Geometry: final body of the model. Coordinates: model frame, mm. Give positions to 0.01 mm unless a question says otherwise; leave off trailing zeros. Order: outer loops, then holes, each group sorted by start corner. A loop starts at its lowest first (then second) coordinate and runs counter-clockwise, first axis right, second up. Notation, with made-up numbers: (17.5, 18.5) - (57.5, 18.5) arc R4 ccw to (57.5, 23.5) - close; hole circle Ø11 at (63, 22). An arc over 180 degrees is marked (long way). Put each result on its own line as item: value. Start each with the question number.
1. Section D-D on z = 3.8. Return the cut outline in (x, y).
2. Ray query, line 1 along Y through (x, z) = (-8.25, 6.6); line 2 along Z through (x, y) = (-6.5, 2.75); line 3 along X through (y, z) = (1.5, 4.55). Return the intervals inside material, ascending. Write a range as from..to.
3. Section A-A on y = 3. Return the cut outline in (x, z).
4. Section B-B on z = 6.6. Return the cut outline in (x, y).
5. Section C-C on x = -7.5. Return the cut outline in (y, z), plus the area to 3 significant figures.
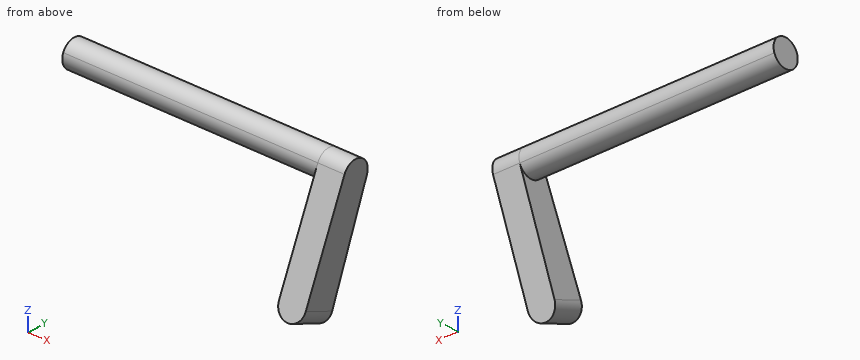
Autodesk Inventor part; units mm, degrees
ref_plane "YZ Plane" through (0, 0, 0) normal (1, 0, 0) x (0, 1, 0)
ref_plane "XZ Plane" through (0, 0, 0) normal (0, 1, 0) x (-1, 0, 0)
ref_plane "XY Plane" through (0, 0, 0) normal (0, 0, 1) x (1, 0, 0)
sketch "Sketch1" plane through (0, 0, 0) normal (1, 0, 0) x (0, 1, 0)
  line L0 (0, 0) -> (2.696, 0)
  line L1 (2.696, 0) -> (2.696, 6.6)
  circle A0 centre (2.696, 6.6) radius 0.5
  line L2 (-0.5, 0.5) -> (0.5, 0.5)
  line L3 (0.5, 0.5) -> (0.5, -0.5)
  line L4 (0.5, -0.5) -> (-0.5, -0.5)
  line L5 (-0.5, -0.5) -> (-0.5, 0.5)
  line L6 (-0.5, 0.5) -> (0.5, -0.5) construction
  line L7 (0.5, 0.5) -> (-0.5, -0.5) construction
  line L8 (0.5, -0.5) -> (3.1627, 6.4205)
  line L9 (-0.5, 0.5) -> (2.2374, 6.7993)
  dimension "d0" = 2.696
  dimension "d1" = 6.6
  dimension "d2" = 1
  dimension "d3" = 1
  dimension "d4" = 1
extrude "Extrusion1" add sketch "Sketch1" along normal blind 1 contours L3 L2 L9 A0 L1 L8 L0 | L3 L4 L5 L2 | L0 L8 L3 | L1 A0 L8 | A0
sketch "Sketch2" plane through (0, 0, 0) normal (-1, 0, 0) x (0, 0, 1)
  line L0 (-0.5, -0.5) -> (0.5, -0.5)
  line L1 (0.5, -0.5) -> (0.5, 0.5)
  line L2 (0.5, 0.5) -> (-0.5, 0.5)
  line L3 (-0.5, 0.5) -> (-0.5, -0.5)
  line L4 (-0.5, -0.5) -> (0.5, 0.5) construction
  line L5 (0.5, -0.5) -> (-0.5, 0.5) construction
  arc A0 (6.7993, 2.2374) -> (6.4205, 3.1627) centre (6.6, 2.696) ccw
  circle A1 centre (6.6, 2.696) radius 0.5
  point P0 (0, 0)
  point P1 (6.4205, 3.1627)
  point P2 (6.7993, 2.2374)
  dimension "d7" = 1
  dimension "d8" = 1
extrude "Extrusion2" add sketch "Sketch2" along normal blind 9.53
sketch "Sketch3" plane through (0, 3.1627, 6.4205) normal (0, 0.9333, -0.3591) x (1, 0, 0)
  line L0 (1, 7.415) -> (1, 0)
  line L1 (1, 0) -> (1, 4)
  line L2 (1, 4) -> (0, 4)
  line L3 (0, -0.0213) -> (0, 6.8408)
  circle A0 centre (0.5, 4) radius 0.5
  line L4 (1, 4) -> (2.2974, 4.6522)
  line L5 (2.2974, 4.6522) -> (2.4132, 8.4295)
  line L6 (2.4132, 8.4295) -> (-8.5006, 8.8849)
  line L7 (-8.5006, 8.8849) -> (-10.8473, 7.9695)
  line L8 (-10.8473, 7.9695) -> (-9.9233, 6.1312)
  line L9 (-9.9233, 6.1312) -> (-3.8147, 5.4684)
  line L10 (-3.8147, 5.4684) -> (0, 4)
  point P0 (0, 7.1279)
  point P1 (1, 4)
  dimension "d11" = 4
extrude "Extrusion3" cut sketch "Sketch3" against normal blind 10 contours A0 L10 L9 L8 L7 L6 L5 L4
properties part number "Radius_Bone1_Joint_UPPER"
Resolved:
1. outline: (0, 0.93) - (1, 0.93) - (1, 2.15) - (0, 2.15) - close
2. line 1: 2.2..3.2
2. line 2: 6.1..7.1
2. line 3: 0..1
3. outline: (-9.53, 6.2) - (0, 6.2) - (0, 6) - (1, 6) - (1, 7) - (-9.53, 7) - close
4. outline: (-9.53, 2.2) - (0, 2.2) - (0, 2.15) - (1, 2.15) - (1, 3.2) - (-9.53, 3.2) - close
5. outline: (2.24, 6.8) arc R0.5 ccw (long way) to (3.16, 6.42) arc R0.5 ccw to start
5. area: 0.785 mm^2
